CAD build for the part. Positions are in the model's coordinates, mm. A direction names the side the tool comes from. Give positions to 0.01 mm unless a question says otherwise; leave off trailing zeros. Loops run counter-clockwise (first coordinate to the right, second up) from the corner with the lowest first, then second, coordinate; pieces in that order, holes last. Notation, with made-up numbers: (80, 61.25) - (138, 61.25) arc R19 ccw to (138, 92.25) - close; hole circle Ø1 at (6.25, 30.25). An arc over 180 degrees is marked (long way). Return JSON: item names as keys, results as strings.
from build123d import *

# Parameters (mm, degrees)
CUT_EXTRUDE1_DEPTH = 39.405728739
SKETCH3_R          = 22.5
SKETCH3_R_2        = 17.5
CUT_EXTRUDE2_DEPTH = 2
CUT_EXTRUDE3_START = -2
SKETCH4_R          = 22.5
SKETCH4_R_2        = 17.5
CUT_EXTRUDE3_DEPTH = 2
FILLET1_R          = 2


with BuildPart() as part:
    # Sketch1 → Revolve1 (revolve)
    with BuildSketch(Plane(origin=(0, 0, 0), x_dir=(0, 0, -1), z_dir=(1, 0, 0)), mode=Mode.PRIVATE) as revolve1_sk:
        Polygon((4.5, 25), (7.5, 25), (7.5, 0), (0, 0), (-7.5, 0), (-7.5, 25), (-4.5, 25), (-2, 19), (2, 19), align=None)
    revolve(revolve1_sk.sketch.rotate(Axis((0, 0, 350.137387165), (0, 0, -1)), 90), axis=Axis((0, 0, 350.137387165), (0, 0, -1)))

    # Sketch2 → Cut-Extrude1 (cut, through all)
    with BuildSketch(Plane.XY.offset(7.5)):
        with BuildLine():
            Line((-2, 9), (2, 9))
            Line((2, 9), (2, 7.745966692))
            ThreePointArc((2, 7.745966692), (0, -8), (-2, 7.745966692))
            Line((-2, 7.745966692), (-2, 9))
        make_face()
    extrude(amount=-CUT_EXTRUDE1_DEPTH, mode=Mode.SUBTRACT)

    # Sketch3 → Cut-Extrude2 (cut)
    with BuildSketch(Plane.XY.offset(7.5)):
        Circle(SKETCH3_R)
        Circle(SKETCH3_R_2, mode=Mode.SUBTRACT)
    extrude(amount=-CUT_EXTRUDE2_DEPTH, mode=Mode.SUBTRACT)

    # Sketch4 → Cut-Extrude3 (cut)
    with BuildSketch(Plane(origin=(0, 0, -7.5), x_dir=(-1, 0, 0), z_dir=(0, 0, -1)).offset(CUT_EXTRUDE3_START)):
        with Locations(Location((0, 0, 0), (0, 0, 180))):
            Circle(SKETCH4_R)
        with Locations(Location((0, 0, 0), (0, 0, 180))):
            Circle(SKETCH4_R_2, mode=Mode.SUBTRACT)
    extrude(amount=CUT_EXTRUDE3_DEPTH, mode=Mode.SUBTRACT)

    # Fillet1
    fillet1_edges = [part.edges().sort_by_distance(p)[0] for p in [
        (-22.5, 0, 5.5),
        (-17.5, 0, 5.5),
        (-22.5, 0, -5.5),
        (-17.5, 0, -5.5),
    ]]
    fillet(fillet1_edges, radius=FILLET1_R - 0.0001)  # a hair under: the kernel refuses the full size


solid = part.part
1. Which spindle directions (+Z, -Z, +X, -X, +Y, -Y) get a long thin tool onto all of the face, cutting with end or side? Do faces 4 (the face through (-4.119, 18.548, -0.028)), 5 (the face through (11, 17, -5.5)), 6 (the face through (22.34, -3.82, 7.5)), 7 (the face through (-22.34, -3.82, -7.5)), 8 (the face through (2, 8, 0)). Say none if no direction does.
Values follow:
{"face 4": "none", "face 5": "-Z", "face 6": "+Z, +X, -X, +Y, -Y", "face 7": "-Z, +X, -X, +Y, -Y", "face 8": "+Z, -Z"}
2. Drill centre lines: probe 1 along Y at (x, z) = (0, 0.5); probe 2 along Y at (x, z) = (-6, 7); probe 3 along Z at (x, y) = (-11, 16). Where is each one in solid material? Low to high.
Values follow:
{"probe 1": "y = -19 to -8, 9 to 19", "probe 2": "y = -24.27 to -21.62, -16.51 to -5.29, 5.29 to 16.51, 21.62 to 24.27", "probe 3": "z = -5.5 to -2.17, 2.17 to 5.5"}
3. Cut at A-A, the plane z = -6.5. Write the cut outline in (x, y).
Values follow:
{"outline": "circle Ø50 at (0, 0); circle Ø35.54 at (0, 0); hole circle Ø44.46 at (0, 0); hole (-2, 7.75) arc R8 ccw (long way) to (2, 7.75) - (2, 9) - (-2, 9) - close"}
4. Drop flat-ended pins along their axis: P1, Ø1.5, axis at x = -0.5, z = -1.5, coming from the +Y side; P2, Ø2, axis at x = -0.5, z = 0.5, coming from the -Y side; P3, Ø6, axis at x = 9.5, z = 3, coming from the -Y side. Give the stop position or say it passes through.
Values follow:
{"P1": "stops at y = 19.59", "P2": "stops at y = -19", "P3": "stops at y = -24.03"}
5. Pull direction Z, two halves, no side cores. Call faces 1 (the face through (8.941, 17.189, -2.156)), 2 (the face through (23.846, -7.509, 5.979)), 3 (the face through (11, -17, 5.5)): +Z half, -Z half, draft (parallel to the pull), parting line (faces both ways), or undercut.
Values follow:
{"face 1": "undercut", "face 2": "draft", "face 3": "+Z half"}
